Here's how the part is built. I have some questions about the finished solid (model axes, mm). A direction names the side the tool comes from. Give positions to 0.01 mm unless a question says otherwise; leave off trailing zeros. Loops run counter-clockwise (first coordinate to the right, second up) from the corner with the lowest first, then second, coordinate; pieces in that order, holes last. Notation, with made-up numbers: (57, 79) - (76, 79) arc R18 cw to (76, 99) - close; hole circle Ø6 at (62, 60.25). An arc over 180 degrees is marked (long way). Return JSON: item names as keys, results as strings. Group by question number.
(1) On a 3-axis mill with a long thin cutter (end or side, diameter ignored), from which of +Z, -Z, +X, -X, +Y, -Y can I reach the whole of each face in a straight line? I mean faces 1 (the flat face through (-15, 10, 0)), 2 (the flat face through (-24, 5, 14)), 3 (the flat face through (-3, 15, 1)). Say none if no direction works.
(2) I need wall thicknesses on probe 1 along Y at (x, z) = (-27.25, 11); probe 2 along Z at (x, y) = (-21.75, 13.5); probe 3 along Z at (x, y) = (-21.5, 16.5). Which ranges of each line are inside material? Lowest first, please. Write a range as [from, to].
(3) If we section it at D-D (z = 2): Please give me the cut outline in (x, y), then the cut area to 3 significant figures.
(4) For P1, Ø6, axis at x = -3.5, y = 6, coming from the +Z side; P2, Ø6, axis at x = -6, y = 9, coming from the +Z side; P3, Ø2.5, axis at y = 9.5, z = 2, coming from the +X side, each with a flat end and sliding along its axis, tell me the tip position at first contact or that it passes through.
(5) If we mould it in two halves opening along Y, with no side actions, what happens to faces 4 (the flat face through (-14.79, 9.86, 9.86)), 5 (the flat face through (-22, 20, 6)), 6 (the flat face through (-22, 0, 6)), 7 (the flat face through (-5, 10, 2))? For each: released by +Y, released by -Y, zero draft, split by the parting line, or undercut.
(6) If we section it at A-A (z = 17.5): Please give me the cut outline in (x, y), then the cut area to 3 significant figures.
(7) If we section it at B-B (x = -4.5): Please give me the cut outline in (y, z), then the cut area to 3 significant figures.
(8) If we section it at C-C (x = -18): Please give me the cut outline in (y, z).
```python
from build123d import *

# Parameters (mm, degrees)
F1_DEPTH = 20
F2_W     = 10
F2_H     = 10
F3_DEPTH = 30.001
F4_W     = 5
F4_H     = 10
F5_DEPTH = 25


with BuildPart() as f1:
    # F0 (on Front) → F1 (new body)
    with BuildSketch(Plane.XZ):
        Polygon((0, 0), (-30, 20), (-30, 0), align=None)
    extrude(amount=-F1_DEPTH)

    # F2 (on face) → F3 (cut, through all)
    with BuildSketch(Plane(origin=(-30, 0, 0), x_dir=(0, -1, 0), z_dir=(-1, 0, 0))):
        with Locations((-10, 15)):
            Rectangle(F2_W, F2_H)
    extrude(amount=-F3_DEPTH, mode=Mode.SUBTRACT)

    # F4 (on Top) → F5 (cut)
    with BuildSketch(Plane.XY):
        with Locations((-2.5, 10)):
            Rectangle(F4_W, F4_H)
    extrude(amount=F5_DEPTH, mode=Mode.SUBTRACT)


solid = f1.part
```
Values:
{
 "1": {"face 1": "-Z, +X, -X, +Y, -Y", "face 2": "+Z, +X, -X", "face 3": "+Z, -Z, +X"},
 "2": {"probe 1": "[0, 5], [15, 20]", "probe 2": "[0, 10]", "probe 3": "[0, 14.33]"},
 "3": {"outline": "(-30, 0) - (-3, 0) - (-3, 5) - (-5, 5) - (-5, 15) - (-3, 15) - (-3, 20) - (-30, 20) - close", "area": "520 mm2"},
 "4": {"P1": "z = 4.33", "P2": "z = 6", "P3": "x = -5"},
 "5": {"face 4": "zero draft", "face 5": "released by +Y", "face 6": "released by -Y", "face 7": "undercut"},
 "6": {"outline": "(-30, 0) - (-26.25, 0) - (-26.25, 5) - (-30, 5) - close; (-30, 15) - (-26.25, 15) - (-26.25, 20) - (-30, 20) - close", "area": "37.5 mm2"},
 "7": {"outline": "(0, 0) - (5, 0) - (5, 3) - (0, 3) - close; (15, 0) - (20, 0) - (20, 3) - (15, 3) - close", "area": "30.0 mm2"},
 "8": {"outline": "(0, 0) - (20, 0) - (20, 12) - (15, 12) - (15, 10) - (5, 10) - (5, 12) - (0, 12) - close"}
}
